For this review, use the dimensioned drawing (mm, ordinates from the lowest corner) and the shaded views. A direction names the side the tool comes from. Give positions to 0.01 mm unless a question says otherwise; leave off trailing zeros. Write each loop counter-clockwise with the first axis right and the second up, starting at its lowest first coordinate (ties: lowest second). Pieces come first, ordered by that corner, then holes.
1) We need section A-A on z = 4.75. Give the number of separate pieces and of enclosed holes in the cut face, and give its area (3 significant figures).
2) For P1, Ø2, axis at x = 9.5, y = 10, coming from the +Z side; P2, Ø5.5, axis at x = 6.35, y = 6.35, coming from the -Z side, all flat-tipped, find the tip position at first contact; note any pin that passes through.
3) We need section D-D on x = 29.5. Give the boundary of the cut face in (y, z) (3 decimals).
4) Machinability: for the marked faces 5 and 6, which of the approach directions +Z, -Z, +X, -X, +Y, -Y give a long, thin tool a straight path to every point of the face, cutting with its end or side? Answer none if there is none.
5) Draft analysis for pull direction X (two halves, no side actions). For the marked faces 1, 2, 3 and 4, state which applies: pulls with the +X half, pulls with the -X half, needs draft (parallel to the pull), parting line crosses it, or undercut.
6) Wall thickness on line 1 along X through (y, z) = (32.5, 5.25); line 2 along Y through (x, z) = (19.05, 5.55); line 3 along X through (y, z) = (21, 5.75): over which ranges is each line inside the solid? List them lowest first.
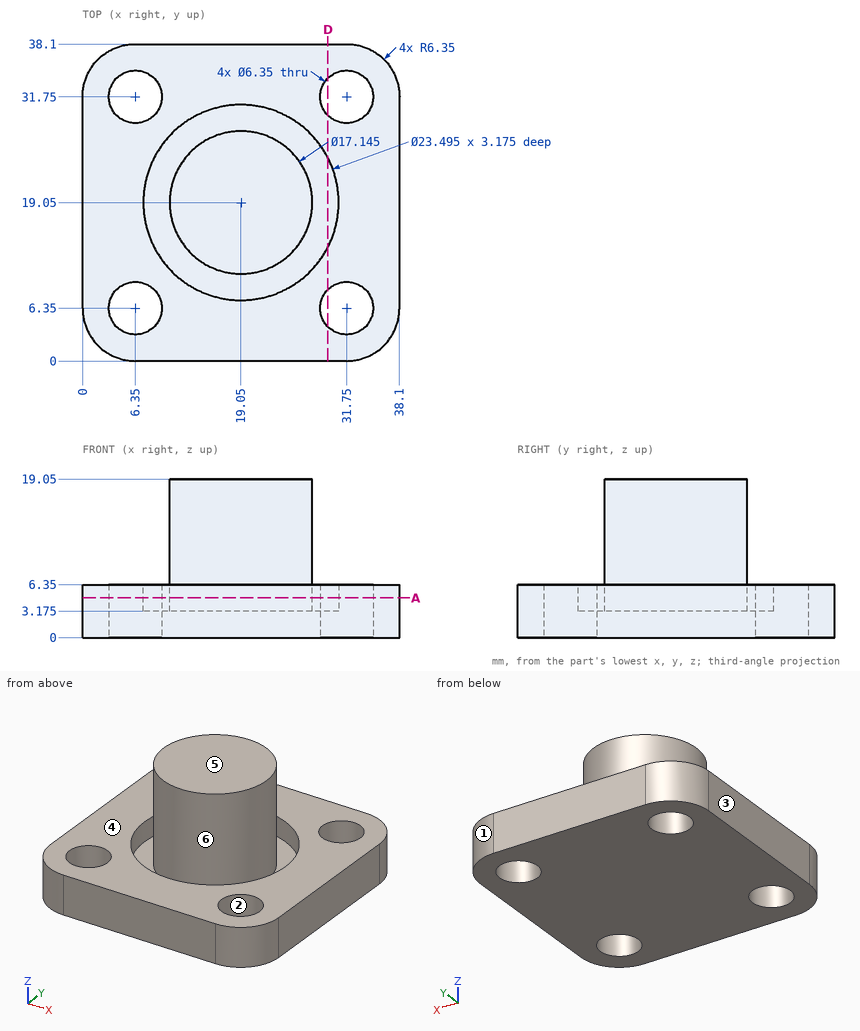
Results list:
1. separate pieces: 2
1. enclosed holes: 5
1. area: 1,090 mm2
2. P1: stops at z = 6.35
2. P2: passes through
3. outline: (0, 0) - (4.11, 0) - (4.11, 6.35) - (0, 6.35) - close; (8.59, 0) - (29.51, 0) - (29.51, 6.35) - (24.417, 6.35) - (24.417, 3.175) - (13.683, 3.175) - (13.683, 6.35) - (8.59, 6.35) - close; (33.99, 0) - (38.1, 0) - (38.1, 6.35) - (33.99, 6.35) - close
4. face 5: +Z, +X, -X, +Y, -Y
4. face 6: +Z
5. face 1: pulls with the +X half
5. face 2: undercut
5. face 3: pulls with the -X half
5. face 4: needs draft
6. line 1: x = 0.04 to 3.26, 9.44 to 28.66, 34.84 to 38.06
6. line 2: y = 0 to 7.3, 10.48 to 27.62, 30.8 to 38.1
6. line 3: x = 0 to 7.47, 10.7 to 27.4, 30.63 to 38.1
